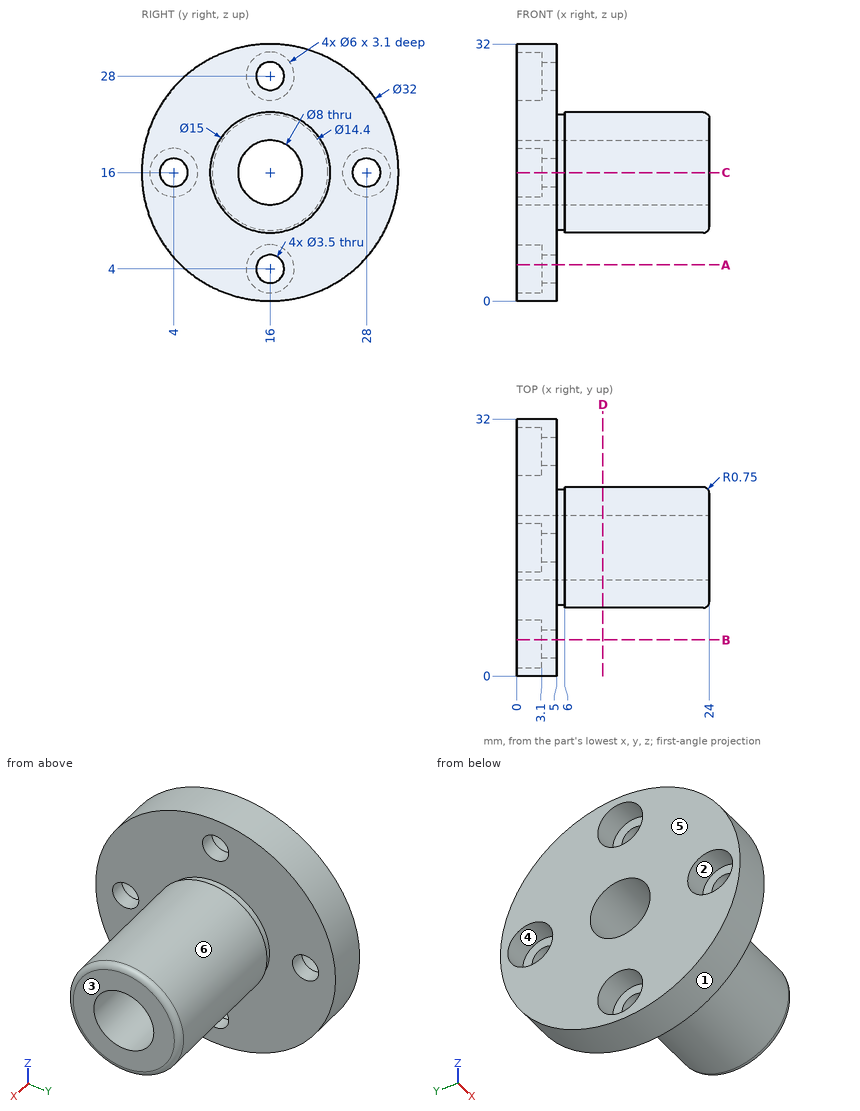
For this review, use the dimensioned drawing (mm, ordinates from the lowest corner) and the shaded views. A direction names the side the tool comes from. Round coordinates to 2 decimals unless told otherwise and drop trailing zeros. Order: outer loops, then holes, each group sorted by start corner. A loop starts at its lowest first (then second) coordinate and runs counter-clockwise, first axis right, second up. Notation, with made-up numbers: (77.5, 38) -> (128.5, 38) arc R13 cw to (128.5, 62) -> close; hole circle Ø8 at (39.5, 39.25). An arc over 180 degrees is marked (long way). One line per item, written item: value. Start each with the question number.
Q1. Mouldability with a two-part tool opening along Y and no side actions: class the marked faces 1, 2 and 3 as released by +Y, released by -Y, zero draft, split by the parting line, or undercut.
Q2. Take a section at D-D (x = 10.75). Write out the cut boundary in (y, z).
Q3. Machinability: for the marked faces 4, 5 and 6, which of the approach directions +Z, -Z, +X, -X, +Y, -Y give a long, thin tool a straight path to every point of the face, cutting with its end or side? Answer none if there is none.
Q4. Take a section at C-C (z = 16). Count the separate pieces of the cut face and the enclosed holes in it, and give its area (3 significant figures).
Q5. Take a section at A-A (z = 4.5). Write out the cut boundary in (x, y), and give its area (3 significant figures).
Q6. Wall thickness on line 1 (Z direction, x = 4.6, y = 16); line 2 (Z direction, x = 2.35, y = 16); line 3 (Z direction, x = 14.5, y = 16): over which ranges is each line inside the solid? List them lowest first.
Q7. Clearance check with flat-ended pins moving along their axes: pin 1 Ø2 at (y, z) = (16, 28) entering from +X; pin 2 Ø12 at (y, z) = (22, 20) entering from -X; pin 3 Ø5.5 at (y, z) = (28, 16) entering from +X; pin 4 Ø5.5 at (y, z) = (16, 28) entering from -X. State where each tip first meets the part, or that it passes through.
Reported:
1. face 1: split by the parting line
1. face 2: undercut
1. face 3: zero draft
2. outline: circle Ø15 at (16, 16); hole circle Ø8 at (16, 16)
3. face 4: -X
3. face 5: +Z, -Z, -X, +Y, -Y
3. face 6: +X
4. separate pieces: 4
4. enclosed holes: 0
4. area: 202 mm2
5. outline: (0, 4.88) -> (5, 4.88) -> (5, 14.32) -> (3.1, 14.32) -> (3.1, 13.04) -> (0, 13.04) -> close; (0, 18.96) -> (3.1, 18.96) -> (3.1, 17.68) -> (5, 17.68) -> (5, 27.12) -> (0, 27.12) -> close
5. area: 86.5 mm2
6. line 1: z = 0 to 2.25, 5.75 to 12, 20 to 26.25, 29.75 to 32
6. line 2: z = 0 to 1, 7 to 12, 20 to 25, 31 to 32
6. line 3: z = 8.5 to 12, 20 to 23.5
7. pin 1: passes through
7. pin 2: stops at x = 0
7. pin 3: stops at x = 5
7. pin 4: stops at x = 3.1
